```python
from build123d import *

# Parameters (mm, degrees)
SKETCH1_W           = 52
SKETCH1_H           = 11.5
BOSS_EXTRUDE1_DEPTH = 0.7
SKETCH2_W           = 52
SKETCH2_H           = 10
BOSS_EXTRUDE2_DEPTH = 0.7
SKETCH3_W           = 46.06
SKETCH3_H           = 5.74
BOSS_EXTRUDE3_DEPTH = 0.215
SKETCH4_W           = 51
SKETCH4_H           = 8.5
BOSS_EXTRUDE4_DEPTH = 0.215


with BuildPart() as part:
    # Sketch1 → Boss-Extrude1 (new body)
    with BuildSketch(Plane.XY):
        Rectangle(SKETCH1_W, SKETCH1_H)
    extrude(amount=BOSS_EXTRUDE1_DEPTH)

    # Sketch2 → Boss-Extrude2 (add)
    with BuildSketch(Plane.XY.offset(0.7)):
        with Locations((0, 0.75)):
            Rectangle(SKETCH2_W, SKETCH2_H)
    extrude(amount=BOSS_EXTRUDE2_DEPTH)

    # Sketch3 → Boss-Extrude3 (add)
    with BuildSketch(Plane.XY.offset(1.4)):
        with Locations((0, 0.75)):
            Rectangle(SKETCH3_W, SKETCH3_H)
    extrude(amount=BOSS_EXTRUDE3_DEPTH)

    # Sketch4 → Boss-Extrude4 (add)
    with BuildSketch(Plane(origin=(0, 0, 0), x_dir=(-1, 0, 0), z_dir=(0, 0, -1))):
        with Locations((0, 0.75)):
            Rectangle(SKETCH4_W, SKETCH4_H)
    extrude(amount=BOSS_EXTRUDE4_DEPTH)


solid = part.part
```
CAD build for the part. Positions are in the model's coordinates, mm. A direction names the side the tool comes from. Coordinates: 2 decimals unless noted, no trailing zeros. Order: outer loops, then holes, each group sorted by start corner. A loop starts at its lowest first (then second) coordinate and runs counter-clockwise, first axis right, second up.
(1) Drill centre lines: L1, parallel to Y at x = -15.5, z = 1.25; L2, parallel to Z at x = -21.5, y = 4 (3 decimals); L3, parallel to Z at x = -3.5, y = -5. Where is each one in solid material? Low to high.
Solution:
L1: y = -4.25 to 5.75
L2: z = -0.215 to 1.4
L3: z = 0 to 0.7
(2) Saw through at B-B, the plane x = -3. Write the cut outline in (y, z) (3 decimals).
Solution:
outline: (-5.75, 0) - (-3.5, 0) - (-3.5, -0.215) - (5, -0.215) - (5, 0) - (5.75, 0) - (5.75, 1.4) - (3.62, 1.4) - (3.62, 1.615) - (-2.12, 1.615) - (-2.12, 1.4) - (-4.25, 1.4) - (-4.25, 0.7) - (-5.75, 0.7) - close
(3) Pin check, flat tip, straight feed: pin 1 Ø1.2 at (x, y) = (3.5, -5) entering from +Z. Stop position of the tip, or through.
Solution:
pin 1: stops at z = 0.7
(4) Saw through at A-A, the plane y = 4.5. Write the cut outline in (x, z) (3 decimals).
Solution:
outline: (-26, 0) - (-25.5, 0) - (-25.5, -0.215) - (25.5, -0.215) - (25.5, 0) - (26, 0) - (26, 1.4) - (-26, 1.4) - close
(5) Which spindle directions (+Z, -Z, +X, -X, +Y, -Y) get a long thin tool onto all of the face, cutting with end or side? Do faces 1 (the face through (0, 5.75, 1)), 2 (the face through (0, -5, 0.7)). Say none if no direction does.
Solution:
face 1: +Z, -Z, +X, -X, +Y
face 2: +Z, +X, -X, -Y
(6) Saw through at D-D, the plane y = -5. Write the cut outline in (x, z).
Solution:
outline: (-26, 0) - (26, 0) - (26, 0.7) - (-26, 0.7) - close
(7) Saw through at C-C, the plane y = -1.25. Write the cut outline in (x, z) (3 decimals).
Solution:
outline: (-26, 0) - (-25.5, 0) - (-25.5, -0.215) - (25.5, -0.215) - (25.5, 0) - (26, 0) - (26, 1.4) - (23.03, 1.4) - (23.03, 1.615) - (-23.03, 1.615) - (-23.03, 1.4) - (-26, 1.4) - close
